Here's the drawing with two shaded views (mm, measured from the low corner). I have some questions. A direction names the side the tool comes from. Coordinates: 2 decimals unless noted, no trailing zeros. Write each loop counter-clockwise with the first axis right and the second up, starting at its lowest first coordinate (ties: lowest second). Pieces come first, ordered by that corner, then holes. Notation, with made-up numbers: (-36.75, 10.5) -> (-26.75, 10.5) arc R13 cw to (-26.75, 22.5) -> close; hole circle Ø2 at (22, 72). An arc over 180 degrees is marked (long way). Put each result on its own line as item: value. Start each with the question number.
Item 1: I want a section at B-B, the plane z = 38.1. List the corners of the cut face in (x, y) for me, then the cut area to 3 significant figures.
Item 2: For pin 1 (3 mm diameter, centred on x = 63.5, z = 36, fed in from -Y); pin 2 (1.5 mm diameter, centred on y = 26.5, z = 57.5, fed in from +X); pin 3 (6.5 mm diameter, centred on x = 44, y = 7.5, fed in from +Z), each with a flat end and sliding along its axis, tell me the tip position at first contact or that it passes through.
Item 3: I need wall thicknesses on line 1 (X direction, y = 21.5, z = 21); line 2 (Y direction, x = 59.5, z = 34.5); line 3 (X direction, y = 5.5, z = 48.5). Which ranges of each line are inside material? Lowest first, please. Write a range as [from, to].
Item 4: I want a section at A-A, the plane y = 50.8. List the corners of the cut face in (x, z) for me, then the cut area to 3 significant figures.
Item 5: On a 3-axis mill with a long thin cutter (end or side, diameter ignored), from which of +Z, -Z, +X, -X, +Y, -Y can I reach the whole of each face in a straight line? I mean the marked faces 1, 2 and 3. Say none if no direction works.
Item 6: I want a section at D-D, the plane z = 8. List the corners of the cut face in (x, y) for me.
Item 7: I want a section at C-C, the plane x = 27. List the corners of the cut face in (y, z) for me.
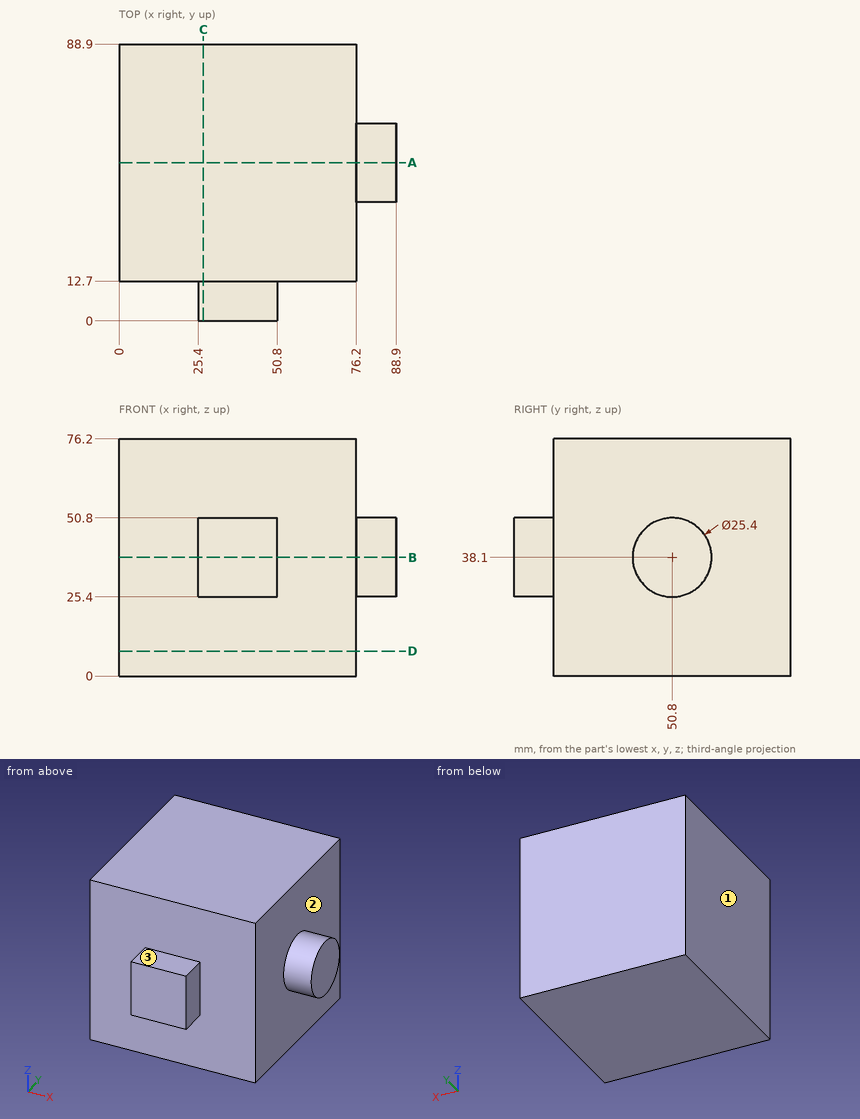
Calculated:
1. outline: (0, 12.7) -> (25.4, 12.7) -> (25.4, 0) -> (50.8, 0) -> (50.8, 12.7) -> (76.2, 12.7) -> (76.2, 38.1) -> (88.9, 38.1) -> (88.9, 63.5) -> (76.2, 63.5) -> (76.2, 88.9) -> (0, 88.9) -> close
1. area: 6,450 mm2
2. pin 1: stops at y = 12.7
2. pin 2: stops at x = 76.2
2. pin 3: stops at z = 50.8
3. line 1: x = [0, 76.2]
3. line 2: y = [12.7, 88.9]
3. line 3: x = [25.4, 50.8]
4. outline: (0, 0) -> (76.2, 0) -> (76.2, 25.4) -> (88.9, 25.4) -> (88.9, 50.8) -> (76.2, 50.8) -> (76.2, 76.2) -> (0, 76.2) -> close
4. area: 6,130 mm2
5. face 1: +Z, -Z, -X, +Y, -Y
5. face 2: +X
5. face 3: +Z, +X, -X, -Y
6. outline: (0, 12.7) -> (76.2, 12.7) -> (76.2, 88.9) -> (0, 88.9) -> close
7. outline: (0, 25.4) -> (12.7, 25.4) -> (12.7, 0) -> (88.9, 0) -> (88.9, 76.2) -> (12.7, 76.2) -> (12.7, 50.8) -> (0, 50.8) -> close
